from build123d import *

# Parameters (mm, degrees)
SKETCH_R        = 60
PAD_DEPTH       = 20
POCKET_DEPTH    = 18
FILLET_R        = 2
FILLET001_R     = 1
CHAMFER_SIZE    = 0.5
FILLET002_R     = 2
FILLET003_R     = 1
CHAMFER001_SIZE = 1


with BuildPart() as part:
    # Sketch → Pad (new body)
    with BuildSketch(Plane.XY):
        with BuildLine():
            ThreePointArc((-73.484692, -15), (58.09475, -47.434165), (0, 75))
            Line((-120, 75), (0, 75))
            ThreePointArc((-120, 75), (-120.393773, 58.298385), (-110.885031, 44.562198))
            ThreePointArc((-73.484692, -15), (-86.775791, 18.177566), (-110.885031, 44.562198))
        make_face()
        Circle(SKETCH_R, mode=Mode.SUBTRACT)
    extrude(amount=PAD_DEPTH)

    # Sketch001 → Pocket (cut)
    with BuildSketch(Plane(origin=(0, 0, 0), x_dir=(1, 0, 0), z_dir=(0, 0, -1))):
        with BuildLine():
            Line((-146.216, -71), (0, -71))
            ThreePointArc((0, -71), (71, 0), (0, 71))
            Line((0, 71), (-146.216, 71))
            Line((-146.216, -71), (-146.216, 71))
        make_face()
    extrude(amount=-POCKET_DEPTH, mode=Mode.SUBTRACT)

    # Fillet
    fillet_edges = [part.edges().sort_by_distance(p)[0] for p in [
        (71, 0, 18),
    ]]
    fillet(fillet_edges, radius=FILLET_R)

    # Fillet001
    fillet001_edges = [part.edges().sort_by_distance(p)[0] for p in [
        (-24.166092, -71, 8),
    ]]
    fillet(fillet001_edges, radius=FILLET001_R)

    # Chamfer
    chamfer_edges = [part.edges().sort_by_distance(p)[0] for p in [
        (-60, 75, 20),
    ]]
    chamfer(chamfer_edges, length=CHAMFER_SIZE)

    # Fillet002
    fillet002_edges = [part.edges().sort_by_distance(p)[0] for p in [
        (-120, 75, 9.75),
    ]]
    fillet(fillet002_edges, radius=FILLET002_R)

    # Fillet003
    fillet003_edges = [part.edges().sort_by_distance(p)[0] for p in [
        (74.49152, -8.718573, 0),
    ]]
    fillet(fillet003_edges, radius=FILLET003_R)

    # Chamfer001
    chamfer001_edges = [part.edges().sort_by_distance(p)[0] for p in [
        (-60, 0, 20),
    ]]
    chamfer(chamfer001_edges, length=CHAMFER001_SIZE)


solid = part.part
Verification items for the finished model (mm, model axes). A direction names the side the tool comes from. Coordinates: 2 decimals unless noted, no trailing zeros. Loops run counter-clockwise (first coordinate to the right, second up) from the corner with the lowest first, then second, coordinate; pieces in that order, holes last. Notation, with made-up numbers: (68, -21) -> (87, -21) arc R29 ccw to (87, 17) -> close; hole circle Ø3 at (27.5, 3.25). An arc over 180 degrees is marked (long way). Answer as a JSON object with one key per item and string values. Group by question number.
Item 1: Scan lines: probe 1 along X at (y, z) = (-53, 19.25); probe 2 along X at (y, z) = (0, 18.45); probe 3 along Y at (x, z) = (-51.5, 14.25). Record each from-to range of solid material in increasing order.
Item 2: Depth check by flat-ended pin: pin 1 (7.5 mm diameter, centred on x = -64.5, z = 7, fed in from -Y); pin 2 (1.5 mm diameter, centred on x = 5, z = 15.5, fed in from -Y); pin 3 (4 mm diameter, centred on x = 36, z = 16, fed in from +Y). Enter the tip coordinate at first touch or a pass-through.
Item 3: Mould release check, pull along Y, two halves, no side actions. Record for faces 1 (the cylindrical face through (73.27, -16.01, 10.12)), 2 (the flat face through (-8, -71, 8)), 3 (the flat face through (-53, 33, 20)), 4 (the cylindrical face through (70.983, 1.561, 8.395)): +Y half, -Y half, draft (parallel to the pull), parting line (faces both ways), or undercut.
Item 4: Tool access check on faces 5 (the cylindrical face through (-59.94, 2.64, 18.49)), 6 (the flat face through (-54, 30, 18)). Record the directions out of +Z, -Z, +X, -X, +Y, -Y that give a thin tool (end or side, any length) a straight path to the whole face; none if there is none.
Item 5: Sectioned sample at A-A on z = 7. Record the boundary of the cut face in (x, y), plus the area to 3 significant figures.
Evaluation:
{
 "1": {"probe 1": "x = -53.07 to -28.65, 28.65 to 53.07", "probe 2": "x = -77.61 to -60, 60 to 75", "probe 3": "y = 71 to 75"},
 "2": {"pin 1": "stops at y = 71", "pin 2": "stops at y = -74.88", "pin 3": "stops at y = 66.85"},
 "3": {"face 1": "parting line", "face 2": "undercut", "face 3": "draft", "face 4": "undercut"},
 "4": {"face 5": "+Z, -Z", "face 6": "-Z, -X"},
 "5": {"outline": "(-120.81, 72.23) arc R1 ccw to (-119.84, 71) -> (0, 71) arc R71 cw to (0, -71) -> (-17.09, -71) arc R1 ccw to (-17.32, -72.97) arc R75 ccw (long way) to (0, 75) -> (-118.54, 75) arc R2 ccw to (-120.46, 73.56) arc R27 ccw to start", "area": "1,460 mm²"}
}
